Could you check a few things on this drawing? It's one solid part, dimensions in mm from its lowest x, y, z. A direction names the side the tool comes from. Round coordinates to 2 decimals unless told otherwise and drop trailing zeros. Order: outer loops, then holes, each group sorted by start corner. A loop starts at its lowest first (then second) coordinate and runs counter-clockwise, first axis right, second up. Notation, with made-up numbers: (43.5, 51) -> (95.5, 51) arc R18 ccw to (95.5, 72) -> close; hole circle Ø7 at (7.25, 63). An arc over 180 degrees is marked (long way). Use a Markdown table: item, result. Add a question column.
(1) If I drill on probe 1 along Y at (x, z) = (29.5, 27) (1 decimal); probe 2 along Z at (x, y) = (50, 2); probe 3 along X at (y, z) = (2, 26) (1 decimal), over which ranges is the centre line in solid material (lowest first)?
(2) On a 3-axis mill with a long thin cutter (end or side, diameter ignored), from which of +Z, -Z, +X, -X, +Y, -Y can I reach the whole of each face in a straight line? I mean the marked faces 1, 2 and 3. Say none if no direction works.
(3) I want a section at B-B, the plane y = 7.75. Please give me the cut outline in (x, z).
(4) I'm going to push flat-ended pins straight in: P1, Ø5, axis at x = 30.16, y = 19.84, coming from the -Z side; P2, Ø6.5, axis at x = 23, y = 9.5, coming from the +Z side; P3, Ø1.5, axis at y = 6, z = 18.5, coming from the -X side. Where does each tip first touch, or does it pass through?
(5) I want a section at A-A, the plane x = 48.5. Please give me the cut outline in (y, z) (1 decimal).
(6) I want a section at D-D, the plane y = 12. Please give me the cut outline in (x, z).
(7) I want a section at C-C, the plane z = 6. Please give me the cut outline in (x, y), then the cut area to 3 significant figures.
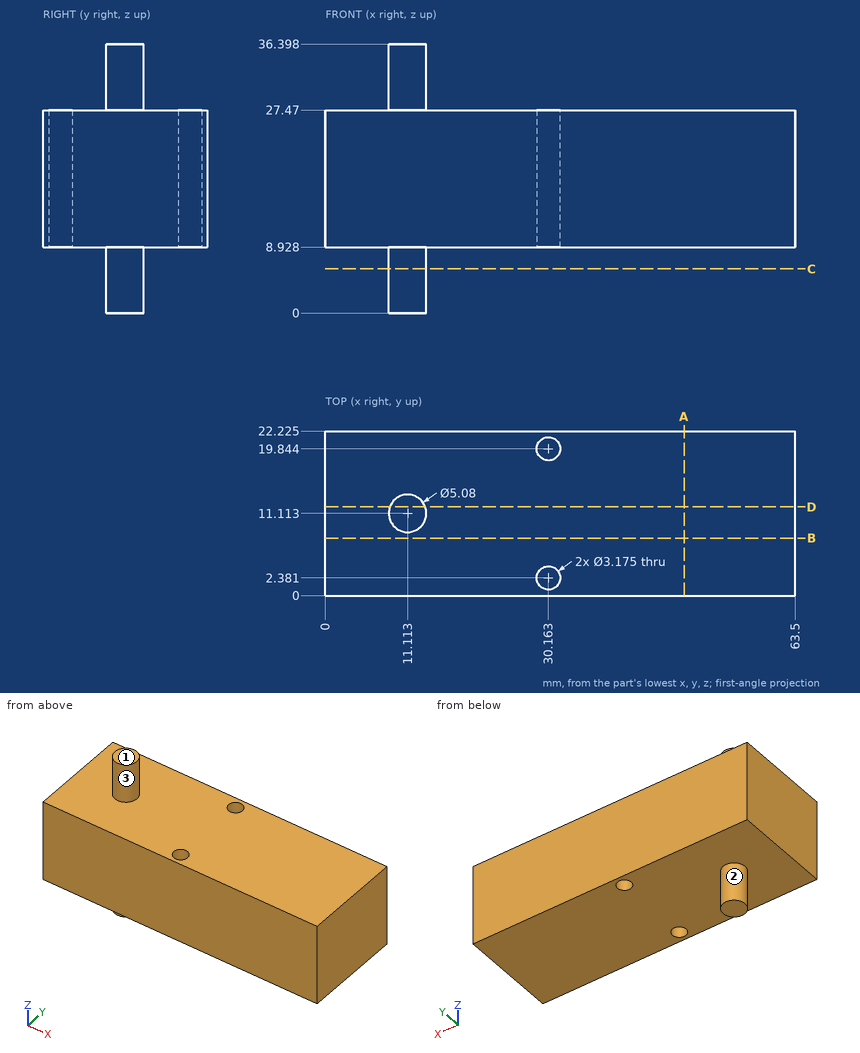
Taken from the geometry:
| question | item | result |
|---|---|---|
| 1 | probe 1 | y = 0 to 0.9, 3.8 to 18.4, 21.3 to 22.2 |
| 1 | probe 2 | z = 8.93 to 27.47 |
| 1 | probe 3 | x = 0 to 28.6, 31.7 to 63.5 |
| 2 | face 1 | +Z, +X, -X, +Y, -Y |
| 2 | face 2 | -Z |
| 2 | face 3 | +Z |
| 3 | outline | (0, 8.93) -> (63.5, 8.93) -> (63.5, 27.47) -> (0, 27.47) -> close |
| 4 | P1 | stops at z = 8.93 |
| 4 | P2 | stops at z = 27.47 |
| 4 | P3 | stops at x = 0 |
| 5 | outline | (0, 8.9) -> (22.2, 8.9) -> (22.2, 27.5) -> (0, 27.5) -> close |
| 6 | outline | (0, 8.93) -> (8.73, 8.93) -> (8.73, 0) -> (13.49, 0) -> (13.49, 8.93) -> (63.5, 8.93) -> (63.5, 27.47) -> (13.49, 27.47) -> (13.49, 36.4) -> (8.73, 36.4) -> (8.73, 27.47) -> (0, 27.47) -> close |
| 7 | outline | circle Ø5.08 at (11.11, 11.11) |
| 7 | area | 20.3 mm2 |
